Autodesk Inventor part; units mm, degrees
ref_plane "YZ Plane" through (0, 0, 0) normal (1, 0, 0) x (0, 1, 0)
ref_plane "XZ Plane" through (0, 0, 0) normal (0, 1, 0) x (-1, 0, 0)
ref_plane "XY Plane" through (0, 0, 0) normal (0, 0, 1) x (1, 0, 0)
ref_plane "Work Plane1" through (0, 0, 0) normal (0, 0, 1) x (1, 0, 0)
sketch "Sketch1" plane through (0, 0, 0) normal (0, 0, 1) x (1, 0, 0)
  circle A0 centre (0, 0) radius 25.9979
  circle A1 centre (-9.4998, -11.0022) radius 2.6601
  circle A2 centre (0.0001, -0.0022) radius 3.8801
  circle A3 centre (0.0001, -0.0022) radius 6.7754
  point P0 (0, 0)
extrude "Extrusion1" add sketch "Sketch1" along normal blind 7 contours A0
sketch "Sketch2" plane through (0, 0, 7) normal (0, 0, 1) x (1, 0, 0)
  line L0 (32.4435, -15.1193) -> (-15.1193, 32.4435)
  line L1 (-15.1193, 32.4435) -> (-32.4435, 15.1193)
  line L2 (-32.4435, 15.1193) -> (15.1193, -32.4435)
  line L3 (15.1193, -32.4435) -> (32.4435, -15.1193)
  line L4 (32.4435, -15.1193) -> (-32.4435, 15.1193) construction
  line L5 (-15.1193, 32.4435) -> (15.1193, -32.4435) construction
  line L6 (32.4435, -15.1193) -> (99.7074, -15.1193) construction
  point P0 (0, 0)
  dimension "d2" = 135
  dimension "d3" = 24.5
extrude "Extrusion2" cut sketch "Sketch2" against normal blind 5
sketch "Sketch3" plane through (0, 0, 7) normal (0, 0, 1) x (1, 0, 0)
  line L0 (-8.3276, -20.7901) -> (-2.5509, -15.0135)
  line L1 (-2.5509, -15.0135) -> (-13.5111, -4.0533)
  line L2 (-19.2877, -9.8299) -> (-13.5111, -4.0533)
  line L3 (-8.3276, -20.7901) -> (-19.2877, -9.8299)
  line L4 (-13.5111, -3.9119) -> (-2.4095, -15.0135)
  line L5 (-2.4095, -15.0135) -> (-8.3276, -20.9315)
  line L6 (-8.3276, -20.9315) -> (-19.4292, -9.8299)
  line L7 (-19.4292, -9.8299) -> (-13.5111, -3.9119)
  line L8 (-8.9176, -8.4066) -> (-24.8767, 7.5526)
  line L9 (-13.4617, -3.8624) -> (-2.4095, -15.0135)
  line L10 (-2.4095, -15.0135) -> (-0.3384, -12.9607)
  line L11 (-0.3384, -12.9607) -> (-11.3905, -1.8096)
  line L12 (-11.3905, -1.8096) -> (-13.4617, -3.8624)
  line L13 (-13.4617, -3.8624) -> (-13.5111, -3.9119)
  line L14 (-8.9176, -8.4066) -> (-24.8767, 7.5526)
  point P0 (0, 0)
  dimension "d6" = 0.1
extrude "Extrusion3" cut sketch "Sketch3" against normal blind 3 contours L3 L2 L1 L0 | L13 L9 L4 | L4 L5 L6 L7 | L9 L12 L11 L10
sketch "Skizze4" plane through (0, 0, 7) normal (0, 0, 1) x (1, 0, 0)
  spline S0 degree 2 poles (24.1427, 2.2394) (24.731, 1.8489) (25.3785, 0.5587) (25.3785, -0.3311) knots 0 0 0 1 2 2 2 construction
  spline S1 degree 2 poles (25.3785, -0.3311) (25.3785, -1.1665) (24.7013, -2.5111) (24.1328, -2.8867) knots 0 0 0 1 2 2 2 construction
  spline S2 degree 2 poles (24.1328, -2.8867) (23.6682, -3.1784) (22.7141, -3.3761) (21.9726, -3.3761) knots 0 0 0 1 2 2 2 construction
  line L0 (21.9726, -3.3761) -> (20.5687, -3.3761) construction
  line L1 (20.5687, -3.3761) -> (20.5687, 2.7239) construction
  line L2 (20.5687, 2.7239) -> (21.9578, 2.7239) construction
  spline S3 degree 2 poles (21.9578, 2.7239) (22.8179, 2.7239) (23.7967, 2.4668) (24.1427, 2.2394) knots 0 0 0 1 2 2 2 construction
  spline S4 degree 2 poles (19.1896, -2.9312) (18.8979, -3.1982) (18.1564, -3.4849) (17.5978, -3.4849) knots 0 0 0 1 2 2 2 construction
  spline S5 degree 2 poles (17.5978, -3.4849) (16.9354, -3.4849) (16.0061, -3.2081) (15.5958, -3.0103) knots 0 0 0 1 2 2 2 construction
  line L3 (15.5958, -3.0103) -> (15.5958, -1.992) construction
  line L4 (15.5958, -1.992) -> (15.6551, -1.992) construction
  spline S6 degree 2 poles (15.6551, -1.992) (16.0555, -2.3677) (17.0689, -2.7829) (17.5385, -2.7829) knots 0 0 0 1 2 2 2 construction
  spline S7 degree 2 poles (17.5385, -2.7829) (18.2108, -2.7829) (18.8979, -2.2243) (18.8979, -1.7646) knots 0 0 0 1 2 2 2 construction
  spline S8 degree 2 poles (18.8979, -1.7646) (18.8979, -1.3988) (18.5371, -0.944) (18.1465, -0.8303) knots 0 0 0 1 2 2 2 construction
  spline S9 degree 2 poles (18.1465, -0.8303) (17.8648, -0.7513) (17.3952, -0.6425) (17.0442, -0.5535) knots 0 0 0 1 2 2 2 construction
  spline S10 degree 2 poles (17.0442, -0.5535) (16.7278, -0.4695) (16.2285, -0.2174) (16.0358, -0.0147) knots 0 0 0 1 2 2 2 construction
  spline S11 degree 2 poles (16.0358, -0.0147) (15.8479, 0.188) (15.6403, 0.7317) (15.6403, 1.0876) knots 0 0 0 1 2 2 2 construction
  spline S12 degree 2 poles (15.6403, 1.0876) (15.6403, 1.8291) (16.797, 2.8326) (17.6918, 2.8326) knots 0 0 0 1 2 2 2 construction
  spline S13 degree 2 poles (17.6918, 2.8326) (18.2059, 2.8326) (19.1154, 2.6299) (19.5059, 2.4372) knots 0 0 0 1 2 2 2 construction
  line L5 (19.5059, 2.4372) -> (19.5059, 1.4683) construction
  line L6 (19.5059, 1.4683) -> (19.4466, 1.4683) construction
  spline S14 degree 2 poles (19.4466, 1.4683) (19.155, 1.7352) (18.2454, 2.1307) (17.7461, 2.1307) knots 0 0 0 1 2 2 2 construction
  spline S15 degree 2 poles (17.7461, 2.1307) (17.1826, 2.1307) (16.4856, 1.6017) (16.4856, 1.1717) knots 0 0 0 1 2 2 2 construction
  spline S16 degree 2 poles (16.4856, 1.1717) (16.4856, 0.7861) (16.8959, 0.3264) (17.2815, 0.2226) knots 0 0 0 1 2 2 2 construction
  spline S17 degree 2 poles (17.2815, 0.2226) (17.5385, 0.1534) (18.285, -0.0246) (18.5321, -0.0987) knots 0 0 0 1 2 2 2 construction
  spline S18 degree 2 poles (18.5321, -0.0987) (19.1599, -0.2915) (19.7432, -1.0676) (19.7432, -1.6361) knots 0 0 0 1 2 2 2 construction
  spline S19 degree 2 poles (19.7432, -1.6361) (19.7432, -1.997) (19.4516, -2.689) (19.1896, -2.9312) knots 0 0 0 1 2 2 2 construction
  circle A0 centre (-9.9998, 17.4978) radius 1.3999 construction
  circle A1 centre (10.0001, 17.4979) radius 1.4 construction
  circle A2 centre (10.0001, -17.5021) radius 1.4 construction
  circle A3 centre (-9.9998, -17.5021) radius 1.4001 construction
  arc A4 (-25.1198, 6.6998) -> (-24.1417, 5.4917) centre (-24.1417, 6.4917) ccw construction
  line L7 (-24.1417, 5.4917) -> (-17.7002, 5.4917) construction
  arc A5 (-15.7002, 3.4917) -> (-17.7002, 5.4917) centre (-17.7002, 3.4917) ccw construction
  line L8 (-15.7002, 3.4917) -> (-15.7002, -4.496) construction
  arc A6 (-17.7002, -6.496) -> (-15.7002, -4.496) centre (-17.7002, -4.496) ccw construction
  line L9 (-17.7002, -6.496) -> (-23.8502, -6.496) construction
  arc A7 (-23.8502, -6.496) -> (-24.8235, -7.7254) centre (-23.8502, -7.496) ccw construction
  arc A8 (-24.8235, -7.7254) -> (-25.1198, 6.6998) centre (0, 0) ccw construction
  circle A9 centre (-9.4998, -11.0022) radius 2.6601 construction
  circle A10 centre (-16.8291, -16.0482) radius 1.4 construction
  circle A11 centre (6.1284, 23.0202) radius 1.4 construction
  circle A12 centre (22.7119, 7.1872) radius 1.4 construction
  circle A13 centre (0.0001, -0.0022) radius 6.5 construction
  point P0 (0, 0)
hole "Bohrung1" at (6.1284, 23.0202, 7) at (22.7119, 7.1872, 7) at (-16.8291, -16.0482, 7) direction (0, 0, -1) diameter 2.8 end through all
properties part number "Matchboxscope_sample_v1"
The model under review builds one solid part; all positions refer to its coordinate system, in mm. A direction names the side the tool comes from. Round coordinates to 2 decimals unless told otherwise and drop trailing zeros. Order: outer loops, then holes, each group sorted by start corner. A loop starts at its lowest first (then second) coordinate and runs counter-clockwise, first axis right, second up. Notation, with made-up numbers: (-32.5, 60.25) -> (-7.5, 60.25) arc R11 ccw to (-7.5, 65.25) -> close; hole circle Ø9 at (11, -32.75). An arc over 180 degrees is marked (long way). One line per item, written item: value. Start each with the question number.
Q1. Take a section at A-A (y = 2.5). Write out the cut boundary in (x, z).
Q2. Clearance check with flat-ended pins moving along their axes: pin 1 Ø6 at (x, y) = (-17, -18) entering from -Z; pin 2 Ø1.5 at (x, y) = (-1, 15) entering from +Z; pin 3 Ø8.5 at (x, y) = (-9.5, -11) entering from +Z. State where each tip first meets the part, or that it passes through.
Q3. Wall thickness on line 1 (X direction, y = 6, z = 1.75); line 2 (Z direction, x = 17.5, y = -8); line 3 (X direction, y = -4, z = 1): over which ranges is each line inside the solid? List them lowest first.
Q4. Take a section at D-D (z = 1). Write out the cut boundary in (x, y), and give its area (3 significant figures).
Q5. Mouldability with a two-part tool opening along Y and no side actions: class faces 6 (the face through (-20.63, 15.82, 1.12)), 7 (the face through (-5.327, -17.931, 5.521)), 8 (the face through (13, 13, 7)) as released by +Y, released by -Y, zero draft, split by the parting line, or undercut.
Q6. Take a section at C-C (z = 5.5). Write out the cut boundary in (x, y).
Q7. Machinability: for faces 1 (the face through (1.829, -19.153, 4.535)), 2 (the face through (-13, -12, 4)), 3 (the face through (-17.009, -0.315, 4.535)), 4 (the face through (24.08, 7.49, 3.45)), 5 (the face through (-16, -14, 7)), which of the approach directions +Z, -Z, +X, -X, +Y, -Y give a long, thin tool a straight path to every point of the face, cutting with its end or side? Answer none if there is none.
Reported:
1. outline: (-25.88, 0) -> (-6.3, 0) -> (-6.3, 2) -> (-19.82, 2) -> (-19.82, 7) -> (-25.88, 7) -> close; (6.3, 0) -> (25.88, 0) -> (25.88, 7) -> (14.82, 7) -> (14.82, 2) -> (6.3, 2) -> close
2. pin 1: stops at z = 0
2. pin 2: stops at z = 2
2. pin 3: stops at z = 4
3. line 1: x = -25.3 to -3.14, 3.14 to 21.97, 23.45 to 25.3
3. line 2: z = 0 to 2
3. line 3: x = -25.69 to -5.47, 5.47 to 25.69
4. outline: circle Ø52 at (0, 0); hole circle Ø2.8 at (-16.83, -16.05); hole circle Ø5.32 at (-9.5, -11); hole circle Ø13.55 at (0, 0); hole circle Ø2.8 at (6.13, 23.02); hole circle Ø2.8 at (22.71, 7.19)
4. area: 1,940 mm2
5. face 6: split by the parting line
5. face 7: undercut
5. face 8: zero draft
6. outline: (-24.88, 7.55) arc R26 ccw to (7.55, -24.88) -> (-2.36, -14.96) -> (-2.41, -15.01) -> (-8.33, -20.93) -> (-19.43, -9.83) -> (-13.51, -3.91) -> (-13.46, -3.86) -> close; (-7.55, 24.88) -> (24.88, -7.55) arc R26 ccw to start; hole circle Ø2.8 at (-16.83, -16.05); hole circle Ø2.8 at (6.13, 23.02); hole circle Ø2.8 at (22.71, 7.19)
7. face 1: +Z, +X
7. face 2: +Z
7. face 3: +Z, +Y
7. face 4: +Z, -Z
7. face 5: +Z, +X, -X, +Y, -Y
